Can you work these out from the model? Positions are in its coordinate system, mm. A direction names the side the tool comes from. Round coordinates to 2 decimals unless told otherwise and drop trailing zeros. Loops run counter-clockwise (first coordinate to the right, second up) from the corner with the lowest first, then second, coordinate; pieces in that order, holes last. Notation, with made-up numbers: M 35.25,14 L 71.25,14 A29 ccw 71.25,39 Z; hole C 78,37.5 d6. An arc over 180 degrees is marked long. Answer as CSV lines item,"result".
from build123d import *

# Parameters (mm, degrees)
BOSS_EXTRUDE1_DEPTH        = 80
BOSS_EXTRUDE1_DEPTH_BACK   = 80
BOSS_EXTRUDE1_2_DEPTH      = 80
BOSS_EXTRUDE1_2_DEPTH_BACK = 80
CUT_EXTRUDE2_DEPTH         = 81
CUT_EXTRUDE2_DEPTH_BACK    = 81
BOSS_EXTRUDE2_DEPTH        = 20
SKETCH6_W                  = 160
SKETCH6_H                  = 160
CUT_EXTRUDE3_DEPTH         = 25
SKETCH7_W                  = 110
SKETCH7_H                  = 110
BOSS_EXTRUDE3_DEPTH        = 25
SKETCH8_R                  = 2
CUT_EXTRUDE4_DEPTH         = 25
SKETCH9_W                  = 47
SKETCH9_H                  = 51.571101879
CUT_EXTRUDE5_DEPTH         = 42
SKETCH10_R                 = 7.5
BOSS_EXTRUDE4_DEPTH        = 10


with BuildPart() as part:
    # Sketch1 → Boss-Extrude1 (new body, two sides)
    with BuildSketch(Plane.XY) as boss_extrude1_sk:
        with BuildLine():
            Line((-80, 0), (80, 0))
            Line((80, 0), (62.763932023, 34.472135955))
            ThreePointArc((62.763932023, 34.472135955), (59.076971234, 38.506508084), (53.819660113, 40))
            Line((53.819660113, 40), (-53.819660113, 40))
            ThreePointArc((-53.819660113, 40), (-59.076971234, 38.506508084), (-62.763932023, 34.472135955))
            Line((-62.763932023, 34.472135955), (-80, 0))
        make_face()
    extrude(amount=BOSS_EXTRUDE1_DEPTH)
    extrude(boss_extrude1_sk.sketch, amount=-BOSS_EXTRUDE1_DEPTH_BACK)


with BuildPart() as body_2:
    # Sketch1 → Boss-Extrude1 2 (new body, two sides)
    with BuildSketch(Plane.XY) as boss_extrude1_2_sk:
        with BuildLine():
            Line((-62.763932023, -54.472135955), (-80, -20))
            Line((-80, -20), (80, -20))
            Line((80, -20), (62.763932023, -54.472135955))
            ThreePointArc((62.763932023, -54.472135955), (59.076971234, -58.506508084), (53.819660113, -60))
            Line((53.819660113, -60), (-53.819660113, -60))
            ThreePointArc((-53.819660113, -60), (-59.076971234, -58.506508084), (-62.763932023, -54.472135955))
        make_face()
    extrude(amount=BOSS_EXTRUDE1_2_DEPTH)
    extrude(boss_extrude1_2_sk.sketch, amount=-BOSS_EXTRUDE1_2_DEPTH_BACK)


with BuildPart() as cut_extrude2_tool:
    # Sketch2 → Cut-Extrude2 (new body, two sides)
    with BuildSketch(Plane(origin=(0, 0, 0), x_dir=(0, 0, -1), z_dir=(1, 0, 0))) as cut_extrude2_sk:
        with BuildLine():
            Line((67.253579514, 22.306235851), (80, 0))
            Line((80, 0), (80, 40))
            Line((80, 40), (36.764044699, 40))
            ThreePointArc((36.764044699, 40), (54.389885267, 35.256134809), (67.253579514, 22.306235851))
        make_face()
        with BuildLine():
            Line((-67.253579514, 22.306235851), (-80, 0))
            Line((-80, 0), (-80, 40))
            Line((-80, 40), (-36.764044699, 40))
            ThreePointArc((-36.764044699, 40), (-54.389885267, 35.256134809), (-67.253579514, 22.306235851))
        make_face()
        with BuildLine():
            Line((80, -60), (36.764044699, -60))
            ThreePointArc((36.764044699, -60), (54.389885267, -55.256134809), (67.253579514, -42.306235851))
            Line((67.253579514, -42.306235851), (80, -20))
            Line((80, -20), (80, -60))
        make_face()
        with BuildLine():
            Line((-67.253579514, -42.306235851), (-80, -20))
            Line((-80, -20), (-80, -60))
            Line((-80, -60), (-36.764044699, -60))
            ThreePointArc((-36.764044699, -60), (-54.389885267, -55.256134809), (-67.253579514, -42.306235851))
        make_face()
    extrude(amount=CUT_EXTRUDE2_DEPTH)
    extrude(cut_extrude2_sk.sketch, amount=-CUT_EXTRUDE2_DEPTH_BACK)


with BuildPart() as part_1:
    add(part.part)

    # Cut-Extrude2: cut by cut_extrude2_tool
    add(cut_extrude2_tool.part, mode=Mode.SUBTRACT)



with BuildPart() as body_2_1:
    add(body_2.part)

    # Cut-Extrude2: cut by cut_extrude2_tool
    add(cut_extrude2_tool.part, mode=Mode.SUBTRACT)


with BuildPart() as part_2:
    add(part_1.part)

    add(body_2_1.part)  # Boss-Extrude2 merges body 2
    # Sketch3 → Boss-Extrude2 (add)
    with BuildSketch(Plane.XZ):
        Polygon((-71.300354804, -80), (71.300354804, -80), (80, -80), (80, 80), (-80, 80), (-80, -80), align=None)
    extrude(amount=BOSS_EXTRUDE2_DEPTH)

    # Sketch6 → Cut-Extrude3 (cut)
    with BuildSketch(Plane(origin=(0, -60, 0), x_dir=(-1, 0, 0), z_dir=(0, -1, 0))):
        Rectangle(SKETCH6_W, SKETCH6_H)
    extrude(amount=-CUT_EXTRUDE3_DEPTH, mode=Mode.SUBTRACT)

    # Sketch7 → Boss-Extrude3 (add)
    with BuildSketch(Plane(origin=(0, -60, 0), x_dir=(-1, 0, 0), z_dir=(0, -1, 0))):
        Rectangle(SKETCH7_W, SKETCH7_H)
    extrude(amount=-BOSS_EXTRUDE3_DEPTH)

    # Sketch8 → Cut-Extrude4 (cut)
    with BuildSketch(Plane(origin=(0, -60, 0), x_dir=(-1, 0, 0), z_dir=(0, -1, 0))):
        with Locations((-37, -37)):
            Circle(SKETCH8_R)
        with Locations((-37, 37)):
            Circle(SKETCH8_R)
        with Locations((37, 37)):
            Circle(SKETCH8_R)
        with Locations((37, -37)):
            Circle(SKETCH8_R)
    extrude(amount=-CUT_EXTRUDE4_DEPTH, mode=Mode.SUBTRACT)

    # Sketch9 → Cut-Extrude5 (cut)
    with BuildSketch(Plane(origin=(80, 0, 0), x_dir=(0, 0, -1), z_dir=(1, 0, 0))):
        with Locations((0, -34.214449061)):
            Rectangle(SKETCH9_W, SKETCH9_H)
    extrude(amount=-CUT_EXTRUDE5_DEPTH, mode=Mode.SUBTRACT)

    # Sketch10 → Boss-Extrude4 (add)
    with BuildSketch(Plane.XZ.offset(8.428898121)):
        with Locations((49.5, 0)):
            Circle(SKETCH10_R)
    extrude(amount=BOSS_EXTRUDE4_DEPTH)


solid = part_2.part
Item 1: If we section it at D-D on x = -37: Write out the boundary of the cut face in (y, z), then the cut area to 3 significant figures.
Output:
outline,"M -60,-55 L -35,-55 L -35,-71.43 L -20,-80 L 0,-80 L 22.31,-67.25 A35.12 ccw 40,-36.76 L 40,36.76 A35.12 ccw 22.31,67.25 L 0,80 L -20,80 L -35,71.43 L -35,55 L -60,55 L -60,39 L -35,39 L -35,35 L -60,35 L -60,-35 L -35,-35 L -35,-39 L -60,-39 Z"
area,"13,400 mm2"
Item 2: On a 3-axis mill with a long thin cutter (end or side, diameter ignored), from which of +Z, -Z, +X, -X, +Y, -Y can I reach the whole of each face in a straight line? I mean faces 4 (the face through (-76, -28, 1)), 5 (the face through (1, -48, 55)), 6 (the face through (1, -48, -55)), 7 (the face through (0.964, 35.385, 54.166)), 8 (the face through (37, -48, -35)). Say none if no direction works.
Output:
face 4,"+Z, -Z, -X, -Y"
face 5,"+Z, +X, -X, -Y"
face 6,"-Z, +X, -X, -Y"
face 7,"+Z, +X, -X, +Y"
face 8,"-Y"
Item 3: Will these pins go through, and if not, where does the flat tip stop? pin 1 (7.5 mm diameter, centred on x = 18.5, y = -53.5, fed in from +Z); pin 2 (20 mm diameter, centred on y = -42, z = 45, fed in from +X); pin 3 (1 mm diameter, centred on x = -15, y = 26, fed in from +Z).
Output:
pin 1,"stops at z = 55"
pin 2,"stops at x = 74"
pin 3,"stops at z = 65.19"
Item 4: If we section it at C-C on z = -17.5: Write out the boundary of the cut face in (x, y).
Output:
outline,"M -80,-20 L -72.5,-35 L -55,-35 L -55,-60 L 38,-60 L 38,-8.43 L 80,-8.43 L 80,0 L 62.76,34.47 A10 ccw 53.82,40 L -53.82,40 A10 ccw -62.76,34.47 L -80,0 Z"
Item 5: If I drill on line 1 along X through (y, z) = (-46, 37); line 2 along X through (y, z) = (-41.5, -36.5), over which ranges is the centre line in solid material (lowest first)? Write a range as from..to.
Output:
line 1,"x = -55..-39, -35..35, 39..55"
line 2,"x = -55..-38.94, -35.06..35.06, 38.94..55"
Item 6: If we section it at B-B on x = -7.5: Write out the boundary of the cut face in (y, z).
Output:
outline,"M -60,-55 L -35,-55 L -35,-71.43 L -20,-80 L 0,-80 L 22.31,-67.25 A35.12 ccw 40,-36.76 L 40,36.76 A35.12 ccw 22.31,67.25 L 0,80 L -20,80 L -35,71.43 L -35,55 L -60,55 Z"
Item 7: We'd pull the mould along Z, two halves only. Please class faces 1 (the face through (-1, -10, -80)), 2 (the face through (49, -18.429, 0)), 3 (the face through (1, -10, 80)): released by +Z, released by -Z, zero draft, split by the parting line, or undercut.
Output:
face 1,"released by -Z"
face 2,"undercut"
face 3,"released by +Z"
Item 8: If we section it at A-A on y = -50: Write out the boundary of the cut face in (x, z), then the cut area to 3 significant figures.
Output:
outline,"M -55,-55 L 55,-55 L 55,-23.5 L 38,-23.5 L 38,23.5 L 55,23.5 L 55,55 L -55,55 Z; hole C -37,-37 d4; hole C -37,37 d4; hole C 37,-37 d4; hole C 37,37 d4"
area,"11,300 mm2"
